from build123d import *

# Parameters (mm, degrees)
EXTRUDE_1_DEPTH      = 12
EXTRUDE_2_REACH      = 35.545
EXTRUDE_2_END_RADIUS = 11.985372339
SKETCH_2_R           = 6
MIRROR_START         = 9.249795062
MIRROR_1_DEPTH       = 2.735782315
MIRROR_1_2_DEPTH     = 0.000409876
CUT_EXTRUDE_1_DEPTH  = 34.545141776
CUT_EXTRUDE_2_DEPTH  = 1
CUT_EXTRUDE_3_DEPTH  = 1
MIRROR_START_2       = 9.250204938
MIRROR_3_DEPTH       = 5.749795062
SKETCH_6_R           = 1.55
CUT_EXTRUDE_4_DEPTH  = 37.245193425
SKETCH_12_W          = 20
SKETCH_12_H          = 12
EXTRUDE_4_DEPTH      = 5
EXTRUDE_5_DEPTH      = 10
EXTRUDE_6_DEPTH      = 12
EXTRUDE_7_DEPTH      = 3.75
EXTRUDE_8_DEPTH      = 3.75
SKETCH_21_R          = 1.5
CUT_EXTRUDE_5_DEPTH  = 3


with BuildPart() as part:
    # 스케치1 → 보스-돌출1 (new body)
    with BuildSketch(Plane.XY):
        with BuildLine():
            Line((14.000204938, 2.291069809), (-13.999795062, 2.291069809))
            Line((-13.999795062, 2.291069809), (-13.999795062, -6.939240191))
            Line((-13.999795062, -6.939240191), (-13.999795062, -15.005030191))
            ThreePointArc((-13.999795062, -15.005030191), (-12.699794, -18.209549332), (-10.647895062, -20.993190191))
            Line((-10.647895062, -20.993190191), (-9.249795062, -20.993190191))
            Line((-9.249795062, -20.993190191), (-9.249795062, -18.61185417))
            ThreePointArc((-9.249795062, -18.61185417), (-10.428409882, -16.897436148), (-11.292795062, -15.005030191))
            ThreePointArc((-11.292795062, -15.005030191), (0.000204938, 0.99497801), (11.293204938, -15.005030191))
            ThreePointArc((11.293204938, -15.005030191), (10.428819757, -16.897436148), (9.250204938, -18.61185417))
            Line((9.250204938, -18.61185417), (9.250204938, -20.993190191))
            Line((9.250204938, -20.993190191), (10.648304938, -20.993190191))
            ThreePointArc((10.648304938, -20.993190191), (12.700203875, -18.209549332), (14.000204938, -15.005030191))
            Line((14.000204938, -15.005030191), (14.000204938, -6.939240191))
            Line((14.000204938, -6.939240191), (14.000204938, 2.291069809))
        make_face()
    extrude(amount=EXTRUDE_1_DEPTH)

    # 보스-돌출2: up to this cylinder (the profile starts inside it)
    extrude_2_end = Plane(origin=(0.000204938, -10.990394329, 6), z_dir=(0, 0, -1)) * Cylinder(EXTRUDE_2_END_RADIUS, 96.060744678, mode=Mode.PRIVATE)
    # 스케치2 → 보스-돌출2 (add, up to the surface)
    with BuildSketch(Plane(origin=(-9.249795062, 0, 0), x_dir=(0, 0, -1), z_dir=(1, 0, 0)), mode=Mode.PRIVATE) as extrude_2_sk1:
        with Locations((-6, -14.993190191)):
            Circle(SKETCH_2_R)
    extrude_2_tool1 = extrude(extrude_2_sk1.sketch, amount=-EXTRUDE_2_REACH, mode=Mode.PRIVATE) & extrude_2_end
    add(extrude_2_tool1.solids().sort_by_distance((-9.249795, -14.99319, 6))[0])

    # 대칭 복사1: read off the stored shape, not the designer's step
    # 대칭 복사1 outline → 대칭 복사1 (add)
    with BuildSketch(Plane.YZ.offset(MIRROR_START)):
        with BuildLine():
            ThreePointArc((-18.61185417, 1.214054847), (-8.993190191, 6), (-18.61185417, 10.785945153))
            Line((-18.61185417, 10.785945153), (-18.61185417, 1.214054847))
        make_face()
    extrude(amount=MIRROR_1_DEPTH)

    # Mirror 1 2 outline → Mirror 1 2 (add)
    with BuildSketch(Plane.YZ.offset(MIRROR_START)):
        with BuildLine():
            Line((-18.61185417, 1.214054847), (-18.61185417, 10.785945153))
            ThreePointArc((-18.61185417, 10.785945153), (-20.993190191, 6), (-18.61185417, 1.214054847))
        make_face()
    extrude(amount=MIRROR_1_2_DEPTH)

    # 스케치3 → 컷-돌출1 (cut, through all)
    with BuildSketch(Plane(origin=(-9.249795062, 0, 0), x_dir=(0, 0, -1), z_dir=(1, 0, 0))):
        with BuildLine():
            Line((-6, -20.993190191), (0, -20.993190191))
            Line((0, -20.993190191), (0, -18.61185417))
            Line((0, -18.61185417), (-1.214054847, -18.61185417))
            ThreePointArc((-1.214054847, -18.61185417), (-3.327172272, -20.364967545), (-6, -20.993190191))
        make_face()
        with BuildLine():
            Line((-12, -20.993190191), (-6, -20.993190191))
            ThreePointArc((-6, -20.993190191), (-8.672827728, -20.364967545), (-10.785945153, -18.61185417))
            Line((-10.785945153, -18.61185417), (-12, -18.61185417))
            Line((-12, -18.61185417), (-12, -20.993190191))
        make_face()
        with BuildLine():
            Line((-12, -18.61185417), (-10.785945153, -18.61185417))
            ThreePointArc((-10.785945153, -18.61185417), (-11.688394805, -16.901635773), (-12, -14.993190191))
            Line((-12, -14.993190191), (-12, -18.61185417))
        make_face()
        with BuildLine():
            Line((-1.214054847, -18.61185417), (0, -18.61185417))
            Line((0, -18.61185417), (0, -14.993190191))
            ThreePointArc((0, -14.993190191), (-0.311605195, -16.901635773), (-1.214054847, -18.61185417))
        make_face()
    extrude(amount=-CUT_EXTRUDE_1_DEPTH, mode=Mode.SUBTRACT)

    # 스케치4 → 컷-돌출2 (cut)
    with BuildSketch(Plane.ZY.offset(13.999795062)):
        Polygon((9.23, -15.005030191), (7.615, -12.207768137), (4.385, -12.207768137), (2.77, -15.005030191), (4.385, -17.802292245), (7.615, -17.802292245), align=None)
    extrude(amount=-CUT_EXTRUDE_2_DEPTH, mode=Mode.SUBTRACT)

    # 스케치5 → 컷-돌출3 (cut)
    with BuildSketch(Plane(origin=(14.000204938, 0, 0), x_dir=(0, 0, -1), z_dir=(1, 0, 0))):
        Polygon((-2.77, -15.005030191), (-4.385, -12.207768137), (-7.615, -12.207768137), (-9.23, -15.005030191), (-7.615, -17.802292245), (-4.385, -17.802292245), align=None)
    extrude(amount=-CUT_EXTRUDE_3_DEPTH, mode=Mode.SUBTRACT)

    # 대칭 복사3: read off the stored shape, not the designer's step
    # 대칭 복사3 outline → 대칭 복사3 (cut)
    with BuildSketch(Plane.YZ.offset(MIRROR_START_2)):
        with BuildLine():
            ThreePointArc((-20.993190191, 6), (-19.235830878, 10.242640687), (-14.993190191, 12))
            Line((-14.993190191, 12), (-20.993190191, 12))
            Line((-20.993190191, 12), (-20.993190191, 6))
        make_face()
        with BuildLine():
            Line((-20.993190191, 0), (-14.993190191, 0))
            ThreePointArc((-14.993190191, 0), (-19.235830878, 1.757359313), (-20.993190191, 6))
            Line((-20.993190191, 6), (-20.993190191, 0))
        make_face()
    extrude(amount=MIRROR_3_DEPTH, mode=Mode.SUBTRACT)

    # 스케치6 → 컷-돌출4 (cut, through all)
    with BuildSketch(Plane.ZY.offset(12.999795062)):
        with Locations((6, -15.005030191)):
            Circle(SKETCH_6_R)
    extrude(amount=-CUT_EXTRUDE_4_DEPTH, mode=Mode.SUBTRACT)

    # 스케치12 → 보스-돌출4 (add)
    with BuildSketch(Plane(origin=(0, 2.291069809, 0), x_dir=(1, 0, 0), z_dir=(0, 1, 0))):
        with Locations((0, -6)):
            Rectangle(SKETCH_12_W, SKETCH_12_H)
    extrude(amount=EXTRUDE_4_DEPTH)

    # 스케치14 → 보스-돌출5 (add, symmetric)
    with BuildSketch(Plane(origin=(0, 0, 0), x_dir=(0, 0, -1), z_dir=(1, 0, 0))):
        Polygon((-12, 7.291069809), (0, 7.291069809), (21.75, 22.291069809), (-33.75, 22.291069809), align=None)
        Polygon((-11.377217009, 9.291069809), (-0.622782991, 9.291069809), (14.602217009, 19.791069809), (-26.602217009, 19.791069809), align=None, mode=Mode.SUBTRACT)
    extrude(amount=EXTRUDE_5_DEPTH, both=True)

    # 스케치15 → 보스-돌출6 (add)
    with BuildSketch(Plane.XY.offset(12)):
        Polygon((-10, 7.291069809), (-13.999795062, 2.291069809), (-10, 2.291069809), align=None)
        Polygon((10, 2.291069809), (14.000204938, 2.291069809), (10, 7.291069809), align=None)
    extrude(amount=-EXTRUDE_6_DEPTH)

    # 스케치19 → 보스-돌출7 (add)
    with BuildSketch(Plane(origin=(6.25, 0, 0), x_dir=(0, 0, -1), z_dir=(1, 0, 0))):
        Polygon((-12, 7.291069809), (-47.823129142, -24.313497594), (-43.022395989, -29.755030191), (30.938064105, -29.755030191), (35.775707613, -24.271660464), (0, 7.291069809), (0, 0.623337928), (28.765859914, -24.755030191), (-40.765859914, -24.755030191), (-12, 0.623337928), align=None)
    extrude_7 = extrude(amount=EXTRUDE_7_DEPTH)

    # 대칭 복사4: 보스-돌출7 across plane
    add(extrude_7.mirror(Plane(origin=(0, 0, 0), x_dir=(0, 0, 1), z_dir=(1, 0, 0))))

    # 스케치20 → 보스-돌출8 (add)
    with BuildSketch(Plane(origin=(10, 0, 0), x_dir=(0, 0, -1), z_dir=(1, 0, 0))):
        Polygon((-12, 7.291069809), (-33.75, 22.291069809), (-33.75, -11.897631945), align=None)
        Polygon((21.75, 22.291069809), (21.75, -11.897631945), (0, 7.291069809), align=None)
    extrude_8 = extrude(amount=-EXTRUDE_8_DEPTH)

    # 대칭 복사5: 보스-돌출8 across plane
    add(extrude_8.mirror(Plane(origin=(0, 0, 0), x_dir=(0, 0, 1), z_dir=(1, 0, 0))))

    # 스케치21 → 컷-돌출5 (cut)
    with BuildSketch(Plane(origin=(0, 22.291069809, 0), x_dir=(1, 0, 0), z_dir=(0, 1, 0))):
        with Locations(Location((5, 9, 0), (0, 0, 270))):
            Circle(SKETCH_21_R)
        with Locations(Location((5, -1, 0), (0, 0, 270))):
            Circle(SKETCH_21_R)
        with Locations(Location((-5, 9, 0), (0, 0, 90))):
            Circle(SKETCH_21_R)
        with Locations(Location((-5, -1, 0), (0, 0, 90))):
            Circle(SKETCH_21_R)
        with Locations(Location((5, -11, 0), (0, 0, 90))):
            Circle(SKETCH_21_R)
        with Locations(Location((5, -21, 0), (0, 0, 90))):
            Circle(SKETCH_21_R)
        with Locations(Location((-5, -21, 0), (0, 0, 270))):
            Circle(SKETCH_21_R)
        with Locations(Location((-5, -11, 0), (0, 0, 270))):
            Circle(SKETCH_21_R)
    extrude(amount=-CUT_EXTRUDE_5_DEPTH, mode=Mode.SUBTRACT)


solid = part.part
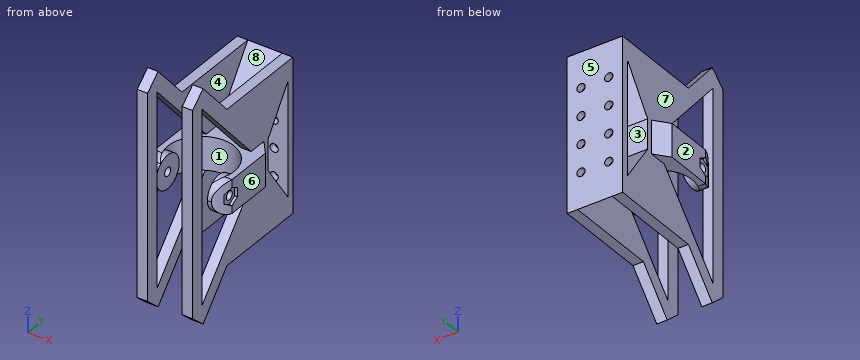
Input: part model. Units: mm. Frame: model coordinates. Face numbers are marked on the shaded views. A direction names the side the tool comes from. Give positions to 0.01 mm unless a question says otherwise; leave off trailing zeros. Write each loop counter-clockwise with the first axis right and the second up, starting at its lowest first coordinate (ties: lowest second). Pieces come first, ordered by that corner, then holes. Notation, with made-up numbers: M 12.5,-6 L 23.5,-6 A26 ccw 23.5,13 Z; hole C 36,-13 d7. An arc over 180 degrees is marked long. Write item = value, one per line. Start each with the question number.
1) Cut plane B-B on y = 16. Return the cut outline in (x, z), then the cut area to 3 significant figures.
2) Draft query along X for the marked faces 6, 7 and 8. Return one class per face: +X half, -X half, draft (parallel to the pull), parting line (faces both ways), or undercut.
3) Reachability of the marked faces 1, 2, 3, 4 and 5 from +Z, -Z, +X, -X, +Y, -Y: full face, straight path, thin tool, end or side. Return the list, or none.
4) Cut plane A-A on z = -20.5. Return the cut outline in (x, y), then the cut area to 3 significant figures.
5) Material intervals for line 1 along X through (y, z) = (21, 11); line 2 along X through (y, z) = (-26.5, -16.5); line 3 along Y through (x, z) = (-9, 20.5), sorted ascending. Write a range as [from, to].
6) First-contact query: pin 1 Ø3 at (y, z) = (4, 24.5) entering from +X; pin 2 Ø6.5 at (x, y) = (-5.5, -4) entering from -Z; pin 3 Ø3.5 at (x, z) = (-5, 11) entering from +Y; pin 4 Ø4 at (x, y) = (-7.5, 9) entering from +Z. Flat tips, straight axial feed; report the tip coordinate or a pass-through.
7) Cut plane D-D on x = -5. Return the cut outline in (y, z), then the cut area to 3 significant figures.
8) Cut plane C-C on x = 1.5. Return the cut outline in (y, z).
Solved:
q1.outline = M -10,-21.75 L -6.25,-21.75 L -6.25,-12.63 L 6.25,-12.63 L 6.25,-21.75 L 10,-21.75 L 10,-9.11 L -10,-9.11 Z; M -10,21.11 L 10,21.11 L 10,33.75 L 6.25,33.75 L 6.25,24.63 L -6.25,24.63 L -6.25,33.75 L -10,33.75 Z
q1.area = 278 mm2
q2.face_6 = +X half
q2.face_7 = -X half
q2.face_8 = undercut
q3.face_1 = none
q3.face_2 = +Z, -Z, -X, +Y, -Y
q3.face_3 = +X, -X
q3.face_4 = -Y
q3.face_5 = +Z, -Z, +X, -X, +Y
q4.outline = M -10,-29.76 L -6.25,-29.76 L -6.25,-24.76 L -10,-24.76 Z; M -10,-17.46 L -6.25,-17.46 L -6.25,21.43 L 6.25,21.43 L 6.25,-17.46 L 10,-17.46 L 10,22.29 L -10,22.29 Z; M 6.25,-29.76 L 10,-29.76 L 10,-24.76 L 6.25,-24.76 Z
q4.area = 346 mm2
q5.line_1 = [-10, -6.5], [-3.5, 3.5], [6.5, 10]
q5.line_2 = [-10, -6.25], [6.25, 10]
q5.line_3 = [-29.76, -24.76], [-6.88, 15.58], [19.79, 22.29]
q6.pin_1 = 10
q6.pin_2 = -21.75
q6.pin_3 = 22.29
q6.pin_4 = 33.75
q7.outline = M -0.1,0 L 7.29,0 L 22.29,-21.75 L 22.29,-10.5 L 19.79,-10.5 L 19.79,-14.6 L 9.29,0.62 L 9.29,11.38 L 19.79,26.6 L 19.79,22.5 L 22.29,22.5 L 22.29,33.75 L 7.29,12 L -0.1,12 Z; M 19.79,-7.5 L 22.29,-7.5 L 22.29,-0.5 L 19.79,-0.5 Z; M 19.79,2.5 L 22.29,2.5 L 22.29,9.5 L 19.79,9.5 Z; M 19.79,12.5 L 22.29,12.5 L 22.29,19.5 L 19.79,19.5 Z
q7.area = 292 mm2
q8.outline = M 0.9,0 L 7.29,0 L 22.29,-21.75 L 22.29,33.75 L 7.29,12 L 0.9,12 Z; hole M 9.29,0.62 L 19.79,-14.6 L 19.79,26.6 L 9.29,11.38 Z
